```python
from build123d import *

# Parameters (mm, degrees)
BOSS_EXTRUDE1_DEPTH = 3.2
SKETCH2_W           = 75.494873271
SKETCH2_H           = 16.574066579
CUT_EXTRUDE1_DEPTH  = 3.2
FILLET1_R           = 0.5
SKETCH3_W           = 8.055614235
SKETCH3_H           = 25.854685688
CUT_EXTRUDE2_DEPTH  = 0.01
SKETCH4_W           = 14.500105624
SKETCH4_H           = 31.26063467
CUT_EXTRUDE3_DEPTH  = 0.01


with BuildPart() as part:
    # Sketch1 → Boss-Extrude1 (new body)
    with BuildSketch(Plane(origin=(0, 0, 0), x_dir=(1, 0, 0), z_dir=(0, 1, 0))):
        with BuildLine():
            ThreePointArc((51.666035076, -4.495071474), (57.875, -2.537392354), (64.083964924, -4.495071474))
            Line((64.083964924, -4.495071474), (64.083964924, -11.181167218))
            ThreePointArc((64.083964924, -11.181167218), (57.875, -9.223488098), (51.666035076, -11.181167218))
            ThreePointArc((51.666035076, -11.181167218), (46.3, -13.686095744), (40.933964924, -11.181167218))
            ThreePointArc((40.933964924, -11.181167218), (34.725, -9.223488098), (28.516035077, -11.181167218))
            ThreePointArc((28.516035077, -11.181167218), (23.15, -13.686095744), (17.783964924, -11.181167218))
            ThreePointArc((17.783964924, -11.181167218), (11.575, -9.223488098), (5.366035077, -11.181167218))
            ThreePointArc((5.366035077, -11.181167218), (0, -13.686095744), (-5.366035076, -11.181167218))
            Line((-5.366035076, -11.181167218), (-5.366035076, -4.495071474))
            ThreePointArc((-5.366035076, -4.495071474), (0, -7), (5.366035076, -4.495071474))
            ThreePointArc((5.366035076, -4.495071474), (11.575, -2.537392354), (17.783964924, -4.495071474))
            ThreePointArc((17.783964924, -4.495071474), (23.15, -7), (28.516035076, -4.495071474))
            ThreePointArc((28.516035076, -4.495071474), (34.725, -2.537392354), (40.933964924, -4.495071474))
            ThreePointArc((40.933964924, -4.495071474), (46.3, -7), (51.666035076, -4.495071474))
        make_face()
    extrude(amount=BOSS_EXTRUDE1_DEPTH)

    # Sketch2 → Cut-Extrude1 (cut)
    with BuildSketch(Plane(origin=(0, 3.2, 0), x_dir=(1, 0, 0), z_dir=(0, 1, 0))):
        with Locations((29.270514079, -6.984979931)):
            Rectangle(SKETCH2_W, SKETCH2_H)
        with BuildLine():
            Line((63.583964924, -10.267724094), (63.583964924, -4.759291488))
            ThreePointArc((63.583964924, -4.759291488), (57.778030808, -3.037847716), (52.005454008, -4.868038061))
            ThreePointArc((52.005454008, -4.868038061), (46.3, -7.5), (40.594545992, -4.868038061))
            ThreePointArc((40.594545992, -4.868038061), (34.725, -3.037392354), (28.855454008, -4.868038061))
            ThreePointArc((28.855454008, -4.868038061), (23.15, -7.5), (17.444545992, -4.868038061))
            ThreePointArc((17.444545992, -4.868038061), (11.575, -3.037392354), (5.705454008, -4.868038061))
            ThreePointArc((5.705454008, -4.868038061), (0.593454673, -7.476483903), (-4.866035076, -5.707162398))
            Line((-4.866035076, -5.707162398), (-4.866035076, -10.995585579))
            ThreePointArc((-4.866035076, -10.995585579), (0.121449449, -13.184961032), (5.023650974, -10.810769172))
            ThreePointArc((5.023650974, -10.810769172), (11.575, -8.723488098), (18.126349026, -10.810769172))
            ThreePointArc((18.126349026, -10.810769172), (23.15, -13.186095744), (28.173650974, -10.810769172))
            ThreePointArc((28.173650974, -10.810769172), (34.725, -8.723488098), (41.276349026, -10.810769172))
            ThreePointArc((41.276349026, -10.810769172), (46.3, -13.186095744), (51.323650974, -10.810769172))
            ThreePointArc((51.323650974, -10.810769172), (57.373874034, -8.734580825), (63.583964924, -10.267724094))
        make_face(mode=Mode.SUBTRACT)
    extrude(amount=-CUT_EXTRUDE1_DEPTH, mode=Mode.SUBTRACT)

    # Fillet1
    fillet1_edges = [part.edges().sort_by_distance(p)[0] for p in [
        (63.583964924, 1.6, 10.267724094),
        (63.583964924, 1.6, 4.759291488),
        (-4.866035076, 1.6, 5.707162398),
        (-4.866035076, 1.6, 10.995585579),
    ]]
    fillet(fillet1_edges, radius=FILLET1_R)

    # Sketch3 → Cut-Extrude2 (cut)
    with BuildSketch(Plane.XZ):
        with Locations((59.701778543, 14.32607503)):
            Rectangle(SKETCH3_W, SKETCH3_H)
    extrude(amount=-CUT_EXTRUDE2_DEPTH, mode=Mode.SUBTRACT)

    # Sketch4 → Cut-Extrude3 (cut)
    with BuildSketch(Plane(origin=(0, 3.2, 0), x_dir=(1, 0, 0), z_dir=(0, 1, 0))):
        with Locations((-5.548696762, 0)):
            Rectangle(SKETCH4_W, SKETCH4_H)
    extrude(amount=-CUT_EXTRUDE3_DEPTH, mode=Mode.SUBTRACT)


solid = part.part
```
Geometry check sheet. Reference: the model listing, model coordinates, mm. Give positions to 0.01 mm unless a question says otherwise; leave off trailing zeros. Write each loop counter-clockwise with the first axis right and the second up, starting at its lowest first coordinate (ties: lowest second). Pieces come first, ordered by that corner, then holes.
1) Release check for a two-part mould opening along X. For faces 1 (the flat face through (26, 0, 8)), 2 (the cylindrical face through (23.2, 1.6, 7.5)), 3 (the flat face through (-4.866, 2, 9)), 4 (the flat face through (63.584, 2, 7)) record: pulls with the +X half, pulls with the -X half, needs draft (parallel to the pull), parting line crosses it, or undercut.
2) Section check B-B, the plane x = 30. Record the boundary of the cut face in (y, z).
3) Section check A-A, the plane y = 1.35. Record the boundary of the cut face in (x, z) (3 decimals).
4) Section check C-C, the plane x = 38.5. Record the boundary of the cut face in (y, z), and give its area (3 significant figures).
5) Gauge pin test, flat ends, axial feed: pin 1 (1.5 mm diameter, centred on x = 45.5, y = 3, fed in from -Z); pin 2 (3.5 mm diameter, centred on x = 61.5, z = 5, fed in from -Y); pin 3 (1.5 mm diameter, centred on x = 21, y = 0.5, fed in from +Z). Record the tip position at first contact, or that the pin passes through.
6) Material ranges on L1, parallel to X at y = 1, z = 6.5; L2, parallel to X at y = 1.4, z = 9.75; L3, parallel to X at y = 2.25, z = 10, recorded low to high.
Computed:
1. face 1: needs draft
1. face 2: undercut
1. face 3: pulls with the -X half
1. face 4: pulls with the +X half
2. outline: (0, 4.18) - (3.2, 4.18) - (3.2, 9.76) - (0, 9.76) - close
3. outline: (-4.866, 6.704) arc R0.5 ccw to (-4.093, 6.285) arc R7.5 cw to (5.705, 4.868) arc R10.325 ccw to (17.445, 4.868) arc R7.5 cw to (28.855, 4.868) arc R10.325 ccw to (40.595, 4.868) arc R7.5 cw to (52.005, 4.868) arc R10.325 ccw to (63.349, 4.608) arc R0.5 ccw to (63.584, 5.032) - (63.584, 9.433) arc R0.5 ccw to (62.864, 9.881) arc R11.325 cw to (51.324, 10.811) arc R6.5 ccw to (41.276, 10.811) arc R11.325 cw to (28.174, 10.811) arc R6.5 ccw to (18.126, 10.811) arc R11.325 cw to (5.024, 10.811) arc R6.5 ccw to (-4.73, 11.145) arc R0.5 ccw to (-4.866, 10.802) - close
4. outline: (0, 3.75) - (3.2, 3.75) - (3.2, 9.37) - (0, 9.37) - close
4. area: 18.0 mm2
5. pin 1: stops at z = 7.34
5. pin 2: stops at y = 0.01
5. pin 3: stops at z = 13.03
6. L1: x = -4.82 to -3.74, 3.74 to 19.41, 26.89 to 42.56, 50.04 to 63.58
6. L2: x = -4.87 to 6.86, 16.29 to 30.01, 39.44 to 53.16, 62.59 to 63.47
6. L3: x = -4.87 to 6.35, 16.8 to 29.5, 39.95 to 52.65
